Verification items for the finished model (mm, model axes). A direction names the side the tool comes from. Give positions to 0.01 mm unless a question says otherwise; leave off trailing zeros. Write each loop counter-clockwise with the first axis right and the second up, starting at its lowest first coordinate (ties: lowest second). Pieces come first, ordered by that corner, then holes. Notation, with made-up numbers: (-12.75, 46) -> (-0.75, 46) arc R25 ccw to (-0.75, 83) -> close; hole circle Ø10 at (16.25, 9). An arc over 180 degrees is marked (long way). Use CSV: the item, a comma, the result in double quotes. Start each with the question number.
```python
from build123d import *

# Parameters (mm, degrees)
SKETCH2_R           = 25
BOSS_EXTRUDE1_DEPTH = 120
SKETCH3_R           = 25
BOSS_EXTRUDE2_DEPTH = 80
SHELL1_OUTLINE_R    = 17.5
SHELL1_DEPTH        = 120
SHELL1_START        = -1e-07
SHELL1_2_OUTLINE_R  = 17.5
SHELL1_2_DEPTH      = 80.0000001
BOSS_EXTRUDE3_START = -5
SKETCH4_R           = 32.5
BOSS_EXTRUDE3_DEPTH = 10
SKETCH5_R           = 17.5
CUT_EXTRUDE1_DEPTH  = 144.809770183


with BuildPart() as part:
    # Sketch2 → Boss-Extrude1 (new body)
    with BuildSketch(Plane(origin=(0, 0, 0), x_dir=(1, 0, 0), z_dir=(0, 1, 0))):
        with Locations(Location((0, 0, 0), (0, 0, 270))):
            Circle(SKETCH2_R)
    extrude(amount=BOSS_EXTRUDE1_DEPTH)

    # Sketch3 → Boss-Extrude2 (add)
    with BuildSketch(Plane.XY):
        with Locations((0, 60)):
            Circle(SKETCH3_R)
    extrude(amount=BOSS_EXTRUDE2_DEPTH)

    # Shell1: read off the stored shape, not the designer's step
    # Shell1 outline → Shell1 (cut)
    with BuildSketch(Plane(origin=(0, 0, 0), x_dir=(1, 0, 0), z_dir=(0, 1, 0))):
        Circle(SHELL1_OUTLINE_R)
    extrude(amount=SHELL1_DEPTH, mode=Mode.SUBTRACT)

    # Shell1 2 outline → Shell1 2 (cut)
    with BuildSketch(Plane.XY.offset(SHELL1_START)):
        with Locations((0, 60)):
            Circle(SHELL1_2_OUTLINE_R)
    extrude(amount=SHELL1_2_DEPTH, mode=Mode.SUBTRACT)

    # Sketch4 → Boss-Extrude3 (add)
    with BuildSketch(Plane.XZ.offset(BOSS_EXTRUDE3_START)):
        with Locations(Location((0, 0, 0), (0, 0, 270))):
            Circle(SKETCH4_R)
    boss_extrude3 = extrude(amount=-BOSS_EXTRUDE3_DEPTH)

    # Mirror1: Boss-Extrude3 across plane
    add(boss_extrude3.mirror(Plane.ZX.offset(60)))

    # Sketch5 → Cut-Extrude1 (cut, through all)
    with BuildSketch(Plane.XZ.offset(-5)):
        with Locations(Location((0, 0, 0), (0, 0, 90))):
            Circle(SKETCH5_R)
    extrude(amount=-CUT_EXTRUDE1_DEPTH, mode=Mode.SUBTRACT)


solid = part.part
```
(1) Set-up check for faces 1 (the face through (-19, 15, -17)), 2 (the face through (7.509, 2.465, 23.846)), 3 (the face through (-19, 115, -17)), 4 (the face through (-17.483, 60.769, 48.329)): record each of +Z, -Z, +X, -X, +Y, -Y from which the full face is reachable in a straight line by a thin tool's end or side.
(2) Section check A-A on x = -28. Record the cut outline in (y, z), then the cut area to 3 significant figures.
(3) Section check C-C on x = -8.5. Give the number of separate pieces and of enclosed holes in the cut face, then the cut area to 3 significant figures.
(4) Thickness scan on line 1 (Y direction, x = 0, z = 39); line 2 (X direction, y = 110, z = 0); line 3 (Z direction, x = -0.5, y = 33) (3 decimals). Record the ranges inside material, lowest first. Write a range as from..to.
(5) Go/stop test with flat-tipped pins: pin 1 (10 mm diameter, centred on y = 60.5, z = 2.5, fed in from +X); pin 2 (4 mm diameter, centred on x = 2.5, z = 55.5, fed in from -Y) (3 decimals); pin 3 (3 mm diameter, centred on y = 44, z = 53.5, fed in from -X); pin 4 (19.5 mm diameter, centred on x = -12.5, z = -2, fed in from -Y). Record where each tip stops, or that it passes through.
(6) Draft check along Y on faces 5 (the face through (-3.255, 84.787, 48.329)), 6 (the face through (-17, 55, 80)), 7 (the face through (-5, 120, -17)), 8 (the face through (-5, 0, -17)). Enter one of: released by +Y, released by -Y, zero draft, split by the parting line, or undercut.
(7) Section check B-B on y = 40. Record the cut outline in (x, z).
Data:
1,face 1,"none"
1,face 2,"-Y"
1,face 3,"+Y"
1,face 4,"+Z"
2,outline,"(5, -16.5) -> (15, -16.5) -> (15, 16.5) -> (5, 16.5) -> close; (105, -16.5) -> (115, -16.5) -> (115, 16.5) -> (105, 16.5) -> close"
2,area,"660 mm2"
3,separate pieces,"3"
3,enclosed holes,"0"
3,area,"2,960 mm2"
4,line 1,"y = 35..42.5, 77.5..85"
4,line 2,"x = -32.5..-17.5, 17.5..32.5"
4,line 3,"z = -24.995..-17.493, 17.493..24.995"
5,pin 1,"stops at x = 25"
5,pin 2,"stops at y = 35.005"
5,pin 3,"stops at x = -20.37"
5,pin 4,"stops at y = 0"
6,face 5,"undercut"
6,face 6,"zero draft"
6,face 7,"released by +Y"
6,face 8,"released by -Y"
7,outline,"(-15, 20) arc R25 ccw (long way) to (15, 20) -> (15, 80) -> (-15, 80) -> close; hole circle Ø35 at (0, 0)"
